```python
from build123d import *

# Parameters (mm, degrees)
EXTRUDE_1_DEPTH     = 16.2
SKETCH_2_R          = 3
EXTRUDE_2_DEPTH     = 8
SKETCH_3_R          = 2
CUT_EXTRUDE_1_DEPTH = 8
SKETCH_4_R          = 8
EXTRUDE_3_DEPTH     = 7
SKETCH_5_R          = 4
EXTRUDE_4_DEPTH     = 30
CUT_EXTRUDE_START   = -16
CUT_EXTRUDE_2_DEPTH = 16
EXTRUDE_5_DEPTH     = 2
SKETCH_9_R          = 18
EXTRUDE_6_DEPTH     = 57.6
FILLET_1_R          = 3
FILLET_2_R          = 1


with BuildPart() as part:
    # 草图1 → 凸台-拉伸1 (new body)
    with BuildSketch(Plane(origin=(0, 0, 0), x_dir=(1, 0, 0), z_dir=(0, 1, 0))):
        with BuildLine():
            Line((-47.75, 30.25), (39.104556615, 30.25))
            ThreePointArc((39.104556615, 30.25), (47.75, 0), (39.104556615, -30.25))
            Line((39.104556615, -30.25), (-47.75, -30.25))
            Line((-47.75, -30.25), (-47.75, 30.25))
        make_face()
    extrude(amount=EXTRUDE_1_DEPTH)

    # 草图2 → 凸台-拉伸2 (add)
    with BuildSketch(Plane(origin=(0, 16.2, 0), x_dir=(1, 0, 0), z_dir=(0, 1, 0))):
        with Locations(Location((-23.75, -20, 0), (0, 0, 90))):
            Circle(SKETCH_2_R)
        with Locations(Location((16.25, -20, 0), (0, 0, 90))):
            Circle(SKETCH_2_R)
        with Locations(Location((16.25, 20, 0), (0, 0, 90))):
            Circle(SKETCH_2_R)
        with Locations(Location((-23.75, 20, 0), (0, 0, 90))):
            Circle(SKETCH_2_R)
    extrude(amount=EXTRUDE_2_DEPTH)

    # 草图3 → 切除-拉伸1 (cut)
    with BuildSketch(Plane(origin=(0, 24.2, 0), x_dir=(1, 0, 0), z_dir=(0, 1, 0))):
        with Locations(Location((-23.75, -20, 0), (0, 0, 270))):
            Circle(SKETCH_3_R)
        with Locations(Location((16.25, -20, 0), (0, 0, 270))):
            Circle(SKETCH_3_R)
        with Locations(Location((16.25, 20, 0), (0, 0, 270))):
            Circle(SKETCH_3_R)
        with Locations(Location((-23.75, 20, 0), (0, 0, 270))):
            Circle(SKETCH_3_R)
    extrude(amount=-CUT_EXTRUDE_1_DEPTH, mode=Mode.SUBTRACT)

    # 草图4 → 凸台-拉伸3 (add)
    with BuildSketch(Plane(origin=(0, 16.2, 0), x_dir=(1, 0, 0), z_dir=(0, 1, 0))):
        with Locations(Location((-23.75, 0, 0), (0, 0, 90))):
            Circle(SKETCH_4_R)
    extrude(amount=EXTRUDE_3_DEPTH)

    # 草图5 → 凸台-拉伸4 (add)
    with BuildSketch(Plane(origin=(0, 23.2, 0), x_dir=(1, 0, 0), z_dir=(0, 1, 0))):
        with Locations(Location((-23.75, 0, 0), (0, 0, 270))):
            Circle(SKETCH_5_R)
    extrude(amount=EXTRUDE_4_DEPTH)

    # 草图6 → 切除-拉伸2 (cut)
    with BuildSketch(Plane(origin=(0, 53.2, 0), x_dir=(1, 0, 0), z_dir=(0, 1, 0)).offset(CUT_EXTRUDE_START)):
        with BuildLine():
            Line((-27.214101615, -2), (-20.285898385, -2))
            ThreePointArc((-20.285898385, -2), (-23.75, -4), (-27.214101615, -2))
        make_face()
    extrude(amount=CUT_EXTRUDE_2_DEPTH, mode=Mode.SUBTRACT)

    # 草图7 → 凸台-拉伸5 (add)
    with BuildSketch(Plane(origin=(0, 16.2, 0), x_dir=(1, 0, 0), z_dir=(0, 1, 0))):
        Polygon((-23.75, -20), (16.25, -20), (32.139613293, -20), (32.139613293, 20), (16.25, 20), (-23.75, 20), align=None)
    extrude(amount=EXTRUDE_5_DEPTH)

    # 草图9 → 凸台-拉伸6 (add)
    with BuildSketch(Plane.XZ):
        with Locations((29.75, 0)):
            Circle(SKETCH_9_R)
    extrude(amount=EXTRUDE_6_DEPTH)

    # 圆角1
    fillet_1_edges = [part.edges().sort_by_distance(p)[0] for p in [
        (11.75, -57.6, 0),
    ]]
    fillet(fillet_1_edges, radius=FILLET_1_R)

    # 圆角2
    fillet_2_edges = [part.edges().sort_by_distance(p)[0] for p in [
        (47.75, 16.2, 0),
        (-4.322721692, 16.2, -30.25),
        (-47.75, 16.2, 0),
        (-4.322721692, 0, -30.25),
        (-4.322721692, 0, 30.25),
        (-47.75, 0, 0),
        (-47.75, 8.1, -30.25),
        (39.104556615, 8.1, -30.25),
        (39.104556615, 8.1, 30.25),
        (-47.75, 8.1, 30.25),
        (-4.322721692, 16.2, 30.25),
    ]]
    fillet(fillet_2_edges, radius=FILLET_2_R)


solid = part.part
```
Geometry check sheet. Reference: the model listing, model coordinates, mm. A direction names the side the tool comes from. Give positions to 0.01 mm unless a question says otherwise; leave off trailing zeros. Order: outer loops, then holes, each group sorted by start corner. A loop starts at its lowest first (then second) coordinate and runs counter-clockwise, first axis right, second up. Notation, with made-up numbers: (77.5, 48) - (118.5, 48) arc R27 cw to (118.5, 84) - close; hole circle Ø1 at (32.25, 24.5). An arc over 180 degrees is marked (long way). Write item = value, one per line. Start each with the question number.
1) Section check B-B (y = 35). Enter the section's corners in (x, z), then the cut area to 3 significant figures.
2) Scan lines: L1, parallel to Z at x = 16, y = 18; L2, parallel to Z at x = 16, y = 21; L3, parallel to X at y = 22, z = 20. Record each from-to range of solid material in increasing order.
3) Section check D-D (x = -38.5). Enter the section's corners in (y, z).
4) Gauge pin test, flat ends, axial feed: pin 1 Ø6.5 at (x, z) = (-24, 20.5) entering from +Y; pin 2 Ø0.6 at (x, y) = (28.5, 17.5) entering from +Z; pin 3 Ø0.6 at (x, z) = (15.5, 21) entering from +Y. Record the tip position at first contact, or that the pin passes through.
5) Access from +Z, -Z, +X, -X, +Y, -Y to the whole of each face (thin tool, end or side, straight path). Record for faces 5 (the flat face through (-22, 23.2, 4)), 6 (the flat face through (-26, 24.2, -20)), 7 (the cylindrical face through (46.919, -26.918, 5.407)).
6) Section check A-A (x = -11). Enter the section's corners in (y, z), then the cut area to 3 significant figures.
7) Draft check along Z on faces 1 (the flat face through (-24, 45, 2)), 2 (the flat face through (-26, 24.2, 20)), 3 (the cylindrical face through (-25.78, 20.14, 22.21)), 4 (the cylindrical face through (47.75, 7.49, -0.44)). Enter one of: released by +Z, released by -Z, zero draft, split by the parting line, or undercut.
8) Section check C-C (x = 29.75). Enter the section's corners in (y, z).
Geometry check:
q1.outline = circle Ø8 at (-23.75, 0)
q1.area = 50.3 mm2
q2.L1 = -22.99 to -21.98, -20 to 20, 21.98 to 22.99
q2.L2 = -22.99 to -21.98, -18.02 to -17.01, 17.01 to 18.02, 21.98 to 22.99
q2.L3 = -26.75 to -25.75, -21.75 to -20.75, 13.25 to 14.25, 18.25 to 19.25
q3.outline = (0, -29.25) arc R1 ccw to (1, -30.25) - (15.2, -30.25) arc R1 ccw to (16.2, -29.25) - (16.2, 29.25) arc R1 ccw to (15.2, 30.25) - (1, 30.25) arc R1 ccw to (0, 29.25) - close
q4.pin_1 = 24.2
q4.pin_2 = 20
q4.pin_3 = 16.2
q5.face_5 = +Y
q5.face_6 = -Z, +X, -X, +Y
q5.face_7 = -Y
q6.outline = (0, -29.25) arc R1 ccw to (1, -30.25) - (15.2, -30.25) arc R1 ccw to (16.2, -29.25) - (16.2, -20) - (18.2, -20) - (18.2, 20) - (16.2, 20) - (16.2, 29.25) arc R1 ccw to (15.2, 30.25) - (1, 30.25) arc R1 ccw to (0, 29.25) - close
q6.area = 1,060 mm2
q7.face_1 = released by +Z
q7.face_2 = zero draft
q7.face_3 = undercut
q7.face_4 = split by the parting line
q8.outline = (-57.6, -15) arc R3 ccw to (-54.6, -18) - (0, -18) - (0, -29.25) arc R1 ccw to (1, -30.25) - (15.2, -30.25) arc R1 ccw to (16.2, -29.25) - (16.2, -20) - (18.2, -20) - (18.2, 20) - (16.2, 20) - (16.2, 29.25) arc R1 ccw to (15.2, 30.25) - (1, 30.25) arc R1 ccw to (0, 29.25) - (0, 18) - (-54.6, 18) arc R3 ccw to (-57.6, 15) - close
